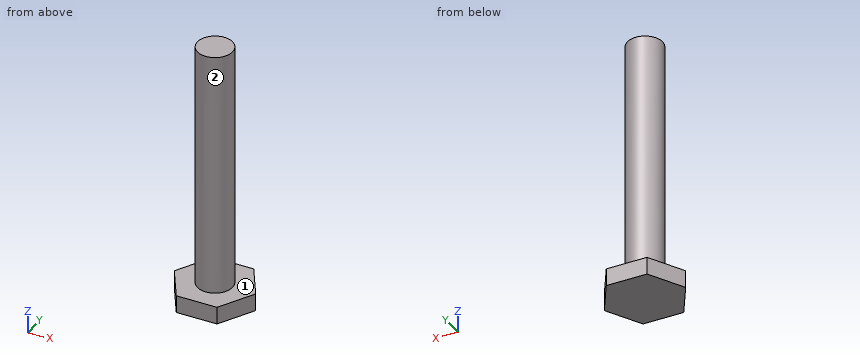
Solid Edge part; units mm, degrees
sketch "Sketch1" plane through (0, 0, 0) normal (0, 0, 1) x (1, 0, 0)
  line L0 (-1.7321, -3) -> (1.7321, -3)
  line L1 (1.7321, -3) -> (3.4641, 0)
  line L2 (3.4641, 0) -> (1.7321, 3)
  line L3 (1.7321, 3) -> (-1.7321, 3)
  line L4 (-1.7321, 3) -> (-3.4641, 0)
  line L5 (-3.4641, 0) -> (-1.7321, -3)
extrude "Protrusion1" add sketch "Sketch1" against normal blind 1.5
sketch "Sketch2" plane through (0, 0, 0) normal (0, 0, 1) x (1, 0, 0)
  circle A0 centre (0, 0) radius 1.5
extrude "ExtrudedProtrusion_2" add sketch "Sketch2" along normal blind 21.2
properties material "Stainless steel"
Check sheet for the modelled part. Datum: model origin and axes. Units: mm. Face numbers are marked on the shaded views. Give positions to 0.01 mm unless a question says otherwise; leave off trailing zeros. Loops run counter-clockwise (first coordinate to the right, second up) from the corner with the lowest first, then second, coordinate; pieces in that order, holes last. Notation, with made-up numbers: M 37.5,54 L 43.5,54 A26 cw 43.5,80 Z; hole C 30,1 d5. An arc over 180 degrees is marked long. Answer in a Markdown table with one row per item.
1) Cross-section at D-D (y = 2.65). Enter the section's corners in (x, z).
Solutions:
| item | result |
|---|---|
| outline | M -1.93,-1.5 L 1.93,-1.5 L 1.93,0 L -1.93,0 Z |
2) Cross-section at C-C (z = 19.5). Enter the section's corners in (x, y), plus the area to 3 significant figures.
Solutions:
| item | result |
|---|---|
| outline | C 0,0 d3 |
| area | 7.07 mm^2 |
3) Depth check by flat-ended pin: pin 1 (1 mm diameter, centred on y = 0.5, z = 14, fed in from +X); pin 2 (1.5 mm diameter, centred on x = 2, y = 0, fed in from +Z); pin 3 (4 mm diameter, centred on x = 2, z = 14, fed in from -Y). Enter the tip coordinate at first touch or a pass-through.
Solutions:
| item | result |
|---|---|
| pin 1 | stops at x = 1.5 |
| pin 2 | stops at z = 21.2 |
| pin 3 | stops at y = -1.5 |
4) Mould release check, pull along X, two halves, no side actions. Record for the marked faces 1 and 2: released by +X, released by -X, zero draft, split by the parting line, or undercut.
Solutions:
| item | result |
|---|---|
| face 1 | zero draft |
| face 2 | split by the parting line |
5) Cross-section at A-A (x = 0). Enter the section's corners in (y, z).
Solutions:
| item | result |
|---|---|
| outline | M -3,-1.5 L 3,-1.5 L 3,0 L 1.5,0 L 1.5,21.2 L -1.5,21.2 L -1.5,0 L -3,0 Z |
6) Cross-section at B-B (y = -0.2). Enter the section's corners in (x, z), plus the area to 3 significant figures.
Solutions:
| item | result |
|---|---|
| outline | M -3.35,-1.5 L 3.35,-1.5 L 3.35,0 L 1.49,0 L 1.49,21.2 L -1.49,21.2 L -1.49,0 L -3.35,0 Z |
| area | 73.1 mm^2 |
7) Thickness scan on line 1 (Z direction, x = -3, y = 0.55); line 2 (X direction, y = -0.9, z = 2.5); line 3 (X direction, y = -0.5, z = 2.5). Record the ranges inside material, lowest first.
Solutions:
| item | result |
|---|---|
| line 1 | z = -1.5 to 0 |
| line 2 | x = -1.2 to 1.2 |
| line 3 | x = -1.41 to 1.41 |
